```python
from build123d import *

# Parameters (mm, degrees)
SKETCH1_R           = 1
BOSS_EXTRUDE1_DEPTH = 5
FILLET1_R           = 5
FILLET2_R           = 5
FILLET3_R           = 5
FILLET4_R           = 3


with BuildPart() as part:
    # Sketch1 → Boss-Extrude1 (new, symmetric)
    with BuildSketch(Plane(origin=(0, 0, 0), x_dir=(1, 0, 0), z_dir=(0, 1, 0))):
        Polygon((0, -60), (-14.281480067, -70), (-64, -70), (-102.5, -32.62), (-102.5, 0), (102.5, 0), (102.5, -32.62), (64, -70), (14.281480067, -70), align=None)
        with Locations(Location((99.5, -8.16, 0), (0, 0, 270))):
            Circle(SKETCH1_R, mode=Mode.SUBTRACT)
        with Locations(Location((99.5, -16.32, 0), (0, 0, 270))):
            Circle(SKETCH1_R, mode=Mode.SUBTRACT)
        with Locations(Location((99.5, -24.48, 0), (0, 0, 270))):
            Circle(SKETCH1_R, mode=Mode.SUBTRACT)
        with Locations(Location((-99.5, -24.48, 0), (0, 0, 90))):
            Circle(SKETCH1_R, mode=Mode.SUBTRACT)
        with Locations(Location((-99.5, -16.32, 0), (0, 0, 90))):
            Circle(SKETCH1_R, mode=Mode.SUBTRACT)
        with Locations(Location((-99.5, -8.16, 0), (0, 0, 90))):
            Circle(SKETCH1_R, mode=Mode.SUBTRACT)
    extrude(amount=BOSS_EXTRUDE1_DEPTH, both=True)

    # Fillet1
    fillet1_edges = [part.edges().sort_by_distance(p)[0] for p in [
        (-14.281480067, 0, 70),
        (14.281480067, 0, 70),
    ]]
    fillet(fillet1_edges, radius=FILLET1_R)

    # Fillet2
    fillet2_edges = [part.edges().sort_by_distance(p)[0] for p in [
        (-64, 0, 70),
        (64, 0, 70),
    ]]
    fillet(fillet2_edges, radius=FILLET2_R)

    # Fillet3
    fillet3_edges = [part.edges().sort_by_distance(p)[0] for p in [
        (-102.5, 0, 32.62),
        (102.5, 0, 32.62),
    ]]
    fillet(fillet3_edges, radius=FILLET3_R)

    # Fillet4
    fillet4_edges = [part.edges().sort_by_distance(p)[0] for p in [
        (-102.5, 0, 0),
        (102.5, 0, 0),
    ]]
    fillet(fillet4_edges, radius=FILLET4_R)

    # Fillet5
    # a fillet whose section is not a circle: 8 mm, written as the material it adds along each edge
    with BuildSketch(Plane(origin=(0, -5, 60), x_dir=(-0.8191520442889911, 0, 0.5735764363510473), z_dir=(0, 1, 0))) as fillet5_piece_1:
        with BuildLine():
            Bezier((5.601660306, 0), (0, 0), (-1.915880661, 5.263838853), weights=[1, 1, 1])
            Line((-1.915880661, 5.263838853), (0, 0))
            Line((0, 0), (5.601660306, 0))
        make_face()
    extrude(amount=10)


solid = part.part
```
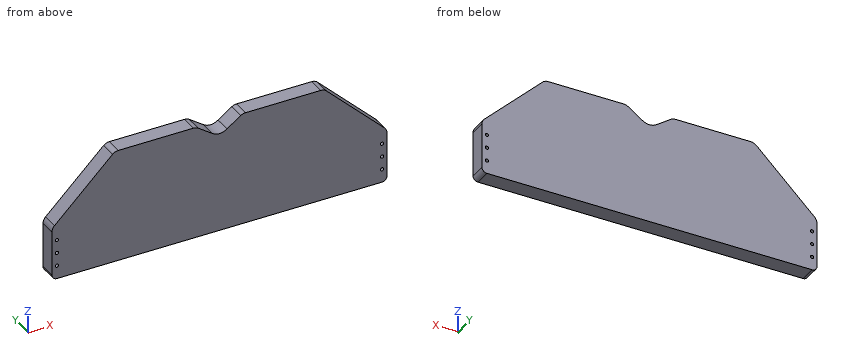
Could you check a few things on this model? Use its own coordinates, in mm. Coordinates: 2 decimals unless noted, no trailing zeros. Write each loop counter-clockwise with the first axis right and the second up, starting at its lowest first coordinate (ties: lowest second). Pieces come first, ordered by that corner, then holes. Notation, with made-up numbers: (74.25, 13) -> (90.25, 13) arc R22 ccw to (90.25, 27) -> close; hole circle Ø7 at (84, 1). An arc over 180 degrees is marked (long way). Write item = value, one per line. Start each with the question number.
(1) I want a section at A-A (y = -1.75). Give the number of separate pieces and of enclosed holes in the cut face, plus the area to 3 significant figures.
(2) I need wall thicknesses on line 1 (X direction, y = 0.5, z = 16.32); line 2 (Z direction, x = -99.5, y = -0.25); line 3 (X direction, y = 2, z = 52.5). Which ranges of each line are inside material? Lowest first, please. Write a range as [from, to].
(3) Will these pins go through, and if not, where does the flat tip stop? pin 1 (3 mm diameter, centred on x = -69.5, y = 0.5, fed in from +Z); pin 2 (1.2 mm diameter, centred on x = -99.5, z = 24.48, fed in from +Y); pin 3 (3 mm diameter, centred on y = -3, z = 36.5, fed in from +X).
(4) I want a section at B-B (z = 47). Please give me the cut outline in (x, y).
(5) I want a section at C-C (x = 70). Please give me the cut outline in (y, z).
Result set:
q1.separate_pieces = 1
q1.enclosed_holes = 6
q1.area = 12,700 mm2
q2.line_1 = [-102.5, -100.5], [-98.5, 98.5], [100.5, 102.5]
q2.line_2 = [0, 7.16], [9.16, 15.32], [17.32, 23.48], [25.48, 35.53]
q2.line_3 = [-82.02, 82.02]
q3.pin_1 = 66.12
q3.pin_2 = through
q3.pin_3 = 100.05
q4.outline = (-87.69, -5) -> (87.69, -5) -> (87.69, 5) -> (-87.69, 5) -> close
q5.outline = (-5, 0) -> (5, 0) -> (5, 64.17) -> (-5, 64.17) -> close
